Design review of the part shown in the three views and the two pictorial views. Dimensions are in mm from the part's minimum x, y and z. A direction names the side the tool comes from. Coordinates: 2 decimals unless noted, no trailing zeros. Order: outer loops, then holes, each group sorted by start corner. A loop starts at its lowest first (then second) coordinate and runs counter-clockwise, first axis right, second up. Notation, with made-up numbers: (-5.5, -20.5) -> (10.5, -20.5) arc R23 ccw to (10.5, -9.5) -> close; hole circle Ø10 at (5.25, 67). An arc over 180 degrees is marked (long way). Write item = value, one per line. Start each with the question number.
1) Consider section A-A on z = 7.25. Give the boundary of the cut face in (x, y) (3 decimals).
2) Consider section C-C on y = 24. Give the boundary of the cut face in (x, z) (3 decimals), and give its area (3 significant figures).
3) Consider section D-D on z = 4. Give the boundary of the cut face in (x, y) (3 decimals), and give its area (3 significant figures).
4) Wall thickness on probe 1 along Z at (x, y) = (15.5, 12.5); probe 2 along Y at (x, z) = (6.5, 10); probe 3 along Y at (x, z) = (17.5, 2.75): over which ranges is each line inside the solid? List them lowest first. Write a range as [from, to].
5) Draft analysis for pull direction Y (two halves, no side actions). For the marked faces 6 and 7, state which applies: +Y half, -Y half, draft (parallel to the pull), parting line (faces both ways), or undercut.
6) Insertion check: pin 1 Ø6 at (y, z) = (6.5, 7) entering from +X (3 decimals); pin 2 Ø8 at (y, z) = (13, 8.5) entering from +X; pin 3 Ø5.5 at (x, y) = (9.5, 14) entering from -Z. Each pin has a flat end and moves straight along its axis. Give the tip position at first contact, or say it passes through.
7) Consider section B-B on x = 13.25. Give the boundary of the cut face in (y, z), and give its area (3 significant figures).
8) Machinability: for the marked faces 1, 2, 3, 4 and 5, which of the approach directions +Z, -Z, +X, -X, +Y, -Y give a long, thin tool a straight path to every point of the face, cutting with its end or side? Answer none if there is none.
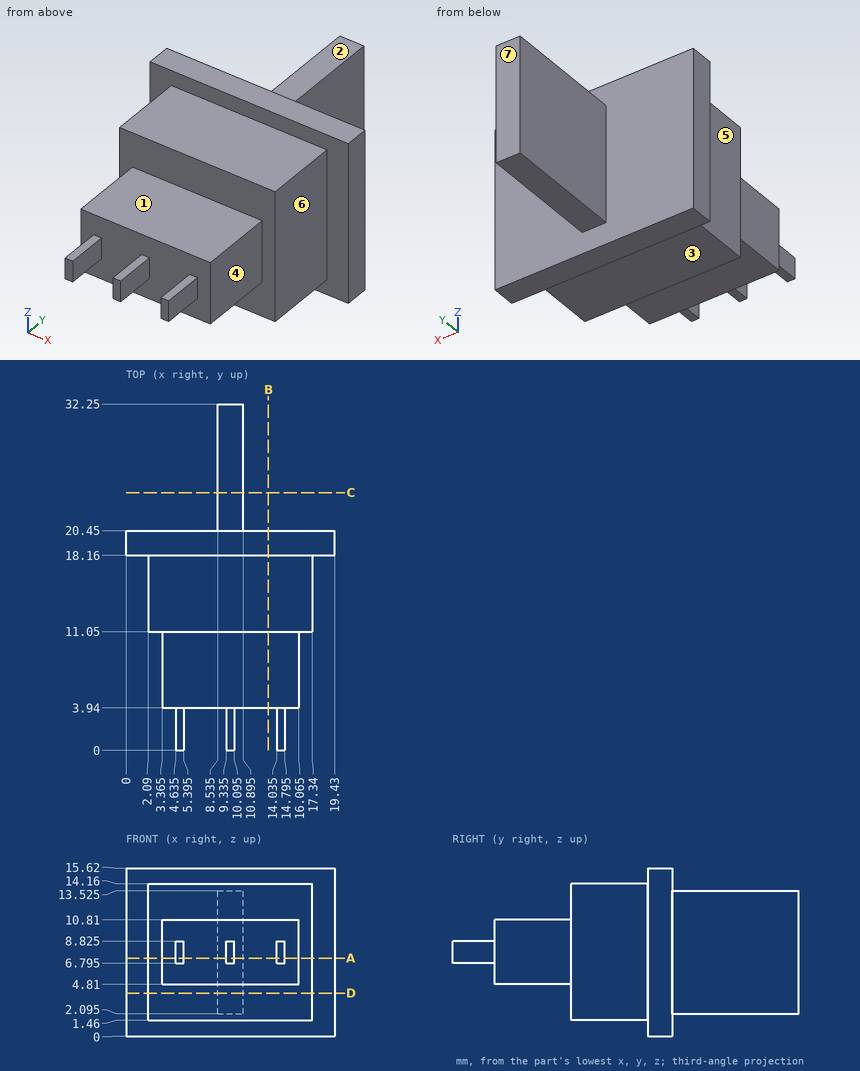
Answer sheet:
q1.outline = (0, 18.16) -> (2.09, 18.16) -> (2.09, 11.05) -> (3.365, 11.05) -> (3.365, 3.94) -> (4.635, 3.94) -> (4.635, 0) -> (5.395, 0) -> (5.395, 3.94) -> (9.335, 3.94) -> (9.335, 0) -> (10.095, 0) -> (10.095, 3.94) -> (14.035, 3.94) -> (14.035, 0) -> (14.795, 0) -> (14.795, 3.94) -> (16.065, 3.94) -> (16.065, 11.05) -> (17.34, 11.05) -> (17.34, 18.16) -> (19.43, 18.16) -> (19.43, 20.45) -> (10.895, 20.45) -> (10.895, 32.25) -> (8.535, 32.25) -> (8.535, 20.45) -> (0, 20.45) -> close
q2.outline = (8.535, 2.095) -> (10.895, 2.095) -> (10.895, 13.525) -> (8.535, 13.525) -> close
q2.area = 27.0 mm2
q3.outline = (0, 18.16) -> (2.09, 18.16) -> (2.09, 11.05) -> (17.34, 11.05) -> (17.34, 18.16) -> (19.43, 18.16) -> (19.43, 20.45) -> (10.895, 20.45) -> (10.895, 32.25) -> (8.535, 32.25) -> (8.535, 20.45) -> (0, 20.45) -> close
q3.area = 181 mm2
q4.probe_1 = [1.46, 14.16]
q4.probe_2 = [3.94, 20.45]
q4.probe_3 = [18.16, 20.45]
q5.face_6 = draft
q5.face_7 = +Y half
q6.pin_1 = 16.065
q6.pin_2 = 17.34
q6.pin_3 = 1.46
q7.outline = (3.94, 4.81) -> (11.05, 4.81) -> (11.05, 1.46) -> (18.16, 1.46) -> (18.16, 0) -> (20.45, 0) -> (20.45, 15.62) -> (18.16, 15.62) -> (18.16, 14.16) -> (11.05, 14.16) -> (11.05, 10.81) -> (3.94, 10.81) -> close
q7.area = 169 mm2
q8.face_1 = +Z, +X, -X, -Y
q8.face_2 = +Z, +X, -X, +Y
q8.face_3 = -Z, +X, -X, -Y
q8.face_4 = +Z, -Z, +X, -Y
q8.face_5 = +Z, -Z, -X, -Y
